Source: CAD feature listing. Evaluate the final solid. Frame: model axes, mm. A direction names the side the tool comes from. Give positions to 0.01 mm unless a question says otherwise; leave off trailing zeros. Write each loop counter-clockwise with the first axis right and the second up, starting at its lowest first coordinate (ties: lowest second). Pieces come first, ordered by that corner, then holes. Notation, with made-up numbers: (36.25, -23.75) -> (91.25, -23.75) arc R19 ccw to (91.25, -11.75) -> close; hole circle Ø3 at (33.5, 5). An arc over 180 degrees is marked (long way). Use one line per item in the form item = value. Start each with the question number.
(1) First-contact query: P1, Ø15, axis at x = 31.5, z = 14, coming from the -Y side; P2, Ø6, axis at x = 27.5, z = 18, coming from the -Y side; P3, Ø2, axis at x = 22.5, z = 11.5, coming from the -Y side. Flat tips, straight axial feed; report the tip coordinate or a pass-through.
(2) Cut plane C-C, the plane z = 25. Count the separate pieces of the cut face and the enclosed holes in it, and give its area (3 significant figures).
(3) Set-up query: faces 5 (the face through (38, 55, 25)), 6 (the face through (132.385, 57.465, 34.751)), 7 (the face through (42, 34, 33)). Return all of +Z, -Z, +X, -X, +Y, -Y with unobstructed straight access to the full face (end or side cutting, diameter ignored); none if empty.
(4) Material intervals for line 1 along Y through (x, z) = (2.5, 25); line 2 along Z through (x, y) = (130, 58); line 3 along Y through (x, z) = (130.5, 37), sorted ascending. Write a range as from..to.
(5) Cut plane B-B, the plane y = 8. Output: boundary loops of the cut face in (x, z).
(6) Draft query along X for faces 1 (the face through (47, 41, 0)), 2 (the face through (47.714, 31.879, 8.381)), 3 (the face through (38.042, 38.089, 8.381)), 4 (the face through (132.31, 57.46, 15.04)). Return one class per face: pulls with the +X half, pulls with the -X half, needs draft (parallel to the pull), parting line crosses it, or undercut.
(7) Cut plane D-D, the plane y = 30.5. Output: boundary loops of the cut face in (x, z), and give its area (3 significant figures).
(8) Cut plane A-A, the plane x = 130. Output: boundary loops of the cut face in (y, z), and give its area (3 significant figures).
Autodesk Fusion 360 part; units mm, degrees
sketch "Sketch1" plane through (0, 0, 0) normal (0, 0, 1) x (1, 0, 0)
  line L0 (0, 0) -> (5, 0)
  line L1 (0, 60) -> (0, 0)
  line L2 (0, 60) -> (150, 60)
  line L3 (150, 60) -> (150, 55)
  line L4 (5, 9.3963) -> (91.6413, 55)
  line L5 (5, 9.3963) -> (91.6413, 55)
  line L6 (70.1715, 55) -> (5, 20.6969)
  line L7 (5, 0) -> (5, 9.3963)
  line L8 (5, 20.6969) -> (5, 55)
  line L9 (150, 55) -> (91.6413, 55)
  line L10 (70.1715, 55) -> (5, 55)
  dimension "d1" = 5
  dimension "d2" = 60
  dimension "d3" = 150
  dimension "d9" = 5
  dimension "d10" = 10
extrude "Extrude1" add sketch "Sketch1" along normal blind 50
sketch "Sketch2" plane through (-2.7881, 5.297, 0) normal (0.4658, -0.8849, 0) x (0, 0, -1)
  line L0 (0, 8.801) -> (0, 106.7113)
  line L1 (0, 106.7113) -> (-50, 106.7113)
  line L2 (-50, 106.7113) -> (-50, 8.801)
  line L3 (-50, 8.801) -> (0, 8.801)
  line L4 (-33, 106.7113) -> (-17, 106.7113)
  line L5 (-17, 106.7113) -> (-17, 8.801)
  line L6 (-17, 8.801) -> (-33, 8.801)
  line L7 (-33, 8.801) -> (-33, 106.7113)
  dimension "d11" = 16
sketch "Sketch3" plane through (-7.4458, 14.1461, 0) normal (-0.4658, 0.8849, 0) x (0, 0, 1)
  line L0 (0, 87.7125) -> (0, 14.0645)
  line L1 (0, 14.0645) -> (50, 14.0645)
  line L2 (50, 14.0645) -> (50, 87.7125)
  line L3 (50, 87.7125) -> (0, 87.7125)
  line L4 (33, 8.801) -> (33, 106.7113)
  line L5 (17, 106.7113) -> (17, 8.801)
extrude "Extrude2" cut sketch "Sketch3" against normal blind 10 contours L1 L3 L4 L5
sketch "Sketch5" plane through (0, 0, 0) normal (0, 1, 0) x (1, 0, 0)
  line L0 (5, -17) -> (91.6413, -17)
  line L1 (91.6413, -17) -> (91.6413, -33)
  line L2 (91.6413, -33) -> (5, -33)
  line L3 (5, -33) -> (5, -17)
  line L4 (5, 0) -> (5, -50)
  line L5 (91.6413, 0) -> (91.6413, -50)
  dimension "d17" = 16
  dimension "d18" = 5
extrude "Extrude3" cut sketch "Sketch5" along normal blind 55
sketch "Sketch4" plane through (5, 0, 0) normal (1, 0, 0) x (0, 0, -1)
  line L0 (0, 0) -> (0, 9.3963)
  line L1 (0, 55) -> (-50, 55)
  line L2 (-50, 55) -> (-50, 20.6969)
  line L3 (-50, 20.6969) -> (-33, 20.6969)
  line L4 (-17, 20.6969) -> (0, 20.6969)
  circle A0 centre (-25, 8) radius 2.5
  circle A1 centre (-25, 24) radius 2.5
  line L5 (-50, 0) -> (0, 0)
  line L6 (0, 9.3963) -> (-17, 9.3963)
  line L7 (-17, 9.3963) -> (-17, 20.6969)
  line L8 (-33, 20.6969) -> (-33, 9.3963)
  line L9 (-33, 9.3963) -> (-50, 9.3963)
  line L10 (-50, 9.3963) -> (-50, 0)
  line L11 (0, 20.6969) -> (0, 55)
  dimension "d14" = 5
  dimension "d22" = 5
  dimension "d23" = 16
extrude "Extrude4" cut sketch "Sketch4" against normal blind 10 contours A0 | A1
sketch "Sketch6" plane through (0, 55, 0) normal (0, -1, 0) x (1, 0, 0)
  line L0 (91.6413, 0) -> (150, 0)
  line L1 (150, 0) -> (150, 50)
  line L2 (150, 50) -> (91.6413, 50)
  line L3 (91.6413, 50) -> (91.6413, 33)
  circle A0 centre (130, 34) radius 2.5
  circle A1 centre (130, 16) radius 2.5
  line L4 (91.6413, 33) -> (70.1715, 33)
  line L5 (70.1715, 33) -> (70.1715, 50)
  line L6 (70.1715, 50) -> (5, 50)
  line L7 (5, 50) -> (5, 0)
  line L8 (5, 0) -> (70.1715, 0)
  line L9 (70.1715, 0) -> (70.1715, 17)
  line L10 (70.1715, 17) -> (91.6413, 17)
  line L11 (91.6413, 17) -> (91.6413, 0)
  dimension "d26" = 5
  dimension "d27" = 20
  dimension "d29" = 5
  dimension "d32" = 16
  dimension "d33" = 16
extrude "Extrude5" cut sketch "Sketch6" against normal blind 10 contours A0 | A1
Geometry says:
q1.P1 = 19.4
q1.P2 = 19.75
q1.P3 = 18.08
q2.separate_pieces = 3
q2.enclosed_holes = 0
q2.area = 975 mm^2
q3.face_5 = +Z, -Z
q3.face_6 = +Y, -Y
q3.face_7 = +X, -Y
q4.line_1 = 0..5.5, 10.5..21.5, 26.5..60
q4.line_2 = 0..13.5, 18.5..31.5, 36.5..50
q4.line_3 = 55..60
q5.outline = (0, 0) -> (5, 0) -> (5, 22.5) -> (0, 22.5) -> close; (0, 27.5) -> (5, 27.5) -> (5, 50) -> (0, 50) -> close
q6.face_1 = needs draft
q6.face_2 = pulls with the +X half
q6.face_3 = undercut
q6.face_4 = undercut
q7.outline = (0, 0) -> (5, 0) -> (5, 50) -> (0, 50) -> close; (23.62, 0) -> (45.09, 0) -> (45.09, 17) -> (23.62, 17) -> close; (23.62, 33) -> (45.09, 33) -> (45.09, 50) -> (23.62, 50) -> close
q7.area = 980 mm^2
q8.outline = (55, 0) -> (60, 0) -> (60, 13.5) -> (55, 13.5) -> close; (55, 18.5) -> (60, 18.5) -> (60, 31.5) -> (55, 31.5) -> close; (55, 36.5) -> (60, 36.5) -> (60, 50) -> (55, 50) -> close
q8.area = 200 mm^2
